Source: CAD feature listing. Evaluate the final solid. Frame: model axes, mm. A direction names the side the tool comes from. Round coordinates to 2 decimals unless told otherwise and drop trailing zeros. Order: outer loops, then holes, each group sorted by start corner. A loop starts at its lowest first (then second) coordinate and runs counter-clockwise, first axis right, second up. Notation, with made-up numbers: M 24,46 L 79,46 A11 cw 79,51 Z; hole C 2,36 d5. An arc over 180 degrees is marked long. Use one line per item in the form item = value. Start each with the question number.
Q1. Section D-D (y = -20). Return the cut outline in (x, z) (3 decimals).
Q2. Section B-B (z = -9.5). Return the cut outline in (x, y) (3 decimals).
Q3. Pull-direction query (X, two-part tool) for faces 3 (the cylindrical face through (12.024, -24.43, -0.86)), 4 (the cylindrical face through (6.8, -11.6, -1.9)), 5 (the flat face through (0, 0, -11)), 6 (the cylindrical face through (6.89, -18.99, 8.54)); classes: pulls with the +X half, pulls with the -X half, needs draft (parallel to the pull), parting line crosses it, or undercut.
Q4. Material intervals for probe 1 along Y at (x, z) = (8, 8.85); probe 2 along Y at (x, z) = (-8, 7.3); probe 3 along Y at (x, z) = (-8, 3), sorted ascending.
Q5. Contact query for flat-ended pins moving along their axis: pin 1 (1.5 mm diameter, centred on x = 8.5, y = -1, fed in from +Z); pin 2 (3.5 mm diameter, centred on x = 8, y = -10.7, fed in from +Z). Output: stop coordinate, or through.
Q6. Reachability of faces 1 (the flat face through (6, 8, 7)), 2 (the flat face through (0, -25, -1)) from +Z, -Z, +X, -X, +Y, -Y: full face, straight path, thin tool, end or side. Return the list, or none.
Q7. Section C-C (x = 8). Give the number of separate pieces and of enclosed holes in the cut face, plus the area to 3 significant figures.
Q8. Section A-A (y = 17.75). Return the cut outline in (x, z) (3 decimals), plus the area to 3 significant figures.
Autodesk Inventor part; units mm, degrees
ref_plane "YZ Plane" through (0, 0, 0) normal (1, 0, 0) x (0, 1, 0)
ref_plane "XZ Plane" through (0, 0, 0) normal (0, 1, 0) x (-1, 0, 0)
ref_plane "XY Plane" through (0, 0, 0) normal (0, 0, 1) x (1, 0, 0)
sketch "Эскиз1" plane through (0, 0, 0) normal (0, 0, 1) x (1, 0, 0)
  line L0 (-12.625, -25) -> (12.625, -25)
  line L1 (12.625, -25) -> (12.625, 25)
  line L2 (12.625, 25) -> (-12.625, 25)
  line L3 (-12.625, 25) -> (-12.625, -25)
  line L4 (-12.625, -25) -> (12.625, 25) construction
  line L5 (12.625, -25) -> (-12.625, 25) construction
  point P0 (0, 0)
  dimension "d0" = 25.25
  dimension "d1" = 50
extrude "Выдавливание1" add sketch "Эскиз1" along normal mid plane 22
fillet "Сопряжение1" radius 2 8 edges at (-12.625, -25, 0) (0, -25, 11) (-12.625, 0, 11) (12.625, 0, 11) (12.625, -25, 0) (0, 25, 11) (12.625, 25, 0) (-12.625, 25, 0)
sketch "Эскиз2" plane through (0, 0, 11) normal (0, 0, 1) x (1, 0, 0)
  circle A0 centre (-8, 17.75) radius 1.25
  circle A1 centre (8, 17.75) radius 1.25
  line L0 (-10.625, 23) -> (10.625, 23)
  point P0 (0, 0)
  dimension "d17" = 5.25
  dimension "d18" = 5.25
extrude "Выдавливание2" cut sketch "Эскиз2" against normal up to surface (22 mm away)
sketch "Эскиз3" plane through (0, 0, 11) normal (0, 0, 1) x (1, 0, 0)
  point P0 (0, 0)
sketch "Эскиз4" plane through (0, 0, 11) normal (0, 0, 1) x (1, 0, 0)
  circle A0 centre (8, 8) radius 1.5
  circle A1 centre (-8, 8) radius 1.5
  line L0 (-8, 8) -> (8, 8) construction
  circle A2 centre (-8, 17.75) radius 1.25 construction
  line L1 (-8, 17.75) -> (-8, 4.7032) construction
  line L2 (10.625, -23) -> (-10.625, -23) construction
  point P0 (0, 0)
  dimension "d7" = 3
  dimension "d8" = 16
  dimension "d16" = 9.75
extrude "Выдавливание3" cut sketch "Эскиз4" against normal up to surface (22 mm away)
sketch "Эскиз5" plane through (0, 0, 11) normal (0, 0, 1) x (1, 0, 0)
  circle A0 centre (8, 8) radius 1.5
  circle A1 centre (8, 8) radius 2.25
  circle A2 centre (-8, 8) radius 1.5
  line L0 (-8, 11.2332) -> (-5.2, 9.6166)
  line L1 (-5.2, 9.6166) -> (-5.2, 6.3834)
  line L2 (-5.2, 6.3834) -> (-8, 4.7668)
  line L3 (-8, 4.7668) -> (-10.8, 6.3834)
  line L4 (-10.8, 6.3834) -> (-10.8, 9.6166)
  line L5 (-10.8, 9.6166) -> (-8, 11.2332)
  point P0 (0, 0)
  dimension "d12" = 4.5
  dimension "d15" = 5.6
extrude "Выдавливание4" cut sketch "Эскиз5" against normal blind 4
sketch "Эскиз6" plane through (0, 0, 11) normal (0, 0, 1) x (1, 0, 0)
  circle A0 centre (-8, -1.3) radius 1.5
  circle A1 centre (8, -1.3) radius 1.5
  circle A2 centre (-8, -20) radius 1.5
  circle A3 centre (8, -20) radius 1.5
  line L0 (-8, -1.3) -> (-8, -20) construction
  line L1 (-8, -1.3) -> (8, -1.3) construction
  line L2 (-8, -20) -> (8, -20) construction
  line L3 (-10.625, -25) -> (10.625, -25)
  line L4 (10.625, -23) -> (-10.625, -23)
  line L5 (0, -23) -> (0, 23) construction
  line L6 (-10.625, 23) -> (10.625, 23)
  line L7 (0, 35) -> (0, -35)
  circle A4 centre (-8, 8) radius 1.5
  point P0 (0, 0)
  point P1 (0, -20)
  dimension "d19" = 3
  dimension "d20" = 16
  dimension "d21" = 16
  dimension "d23" = 5
  dimension "d40" = 9.3
extrude "Выдавливание5" cut sketch "Эскиз6" against normal blind 5 contours A0 | A1 | A2 | A3
sketch "Эскиз7" plane through (0, 0, 11) normal (0, 0, 1) x (1, 0, 0)
  circle A0 centre (-8, -20) radius 1.5
  circle A1 centre (-8, -1.3) radius 1.5
  line L0 (-8, -20) -> (-8, -1.3) construction
  circle A2 centre (8, -20) radius 1.5
  circle A3 centre (8, -1.3) radius 1.5
  line L1 (8, -20) -> (8, -1.3) construction
  circle A4 centre (8, -10.7) radius 2.25
  line L2 (-10.8, -9.0834) -> (-8, -7.4668)
  line L3 (-8, -7.4668) -> (-5.2, -9.0834)
  line L4 (-5.2, -9.0834) -> (-5.2, -12.3166)
  line L5 (-5.2, -12.3166) -> (-8, -13.9332)
  line L6 (-8, -13.9332) -> (-10.8, -12.3166)
  line L7 (-10.8, -12.3166) -> (-10.8, -9.0834)
  circle A5 centre (-8, -10.7) radius 1.5
  circle A6 centre (8, -10.7) radius 1.5
  point P0 (0, 0)
  dimension "d28" = 4.5
  dimension "d29" = 5.6
  dimension "d35" = 3
  dimension "d41" = 9.3
  dimension "d42" = 9.3
extrude "Выдавливание8" cut sketch "Эскиз7" against normal blind 4 contours A4 | L2 L3 L4 L5 L6 L7
sketch "Эскиз9" plane through (0, 0, 11) normal (0, 0, 1) x (1, 0, 0)
  circle A0 centre (-8, -10.7) radius 1.5
  circle A1 centre (8, -10.7) radius 1.5
  point P0 (0, 0)
extrude "Выдавливание9" cut sketch "Эскиз9" against normal up to surface (22 mm away)
properties part number "крепление петли хвоста"
Results list:
q1.outline = M -12.625,-11 L 12.625,-11 L 12.625,9 A2 ccw 10.625,11 L 9.5,11 L 9.5,6 L 6.5,6 L 6.5,11 L -6.5,11 L -6.5,6 L -9.5,6 L -9.5,11 L -10.625,11 A2 ccw -12.625,9 Z
q2.outline = M -12.625,-23 A2 ccw -10.625,-25 L 10.625,-25 A2 ccw 12.625,-23 L 12.625,23 A2 ccw 10.625,25 L -10.625,25 A2 ccw -12.625,23 Z; hole C -8,-10.7 d3; hole C -8,8 d3; hole C -8,17.75 d2.5; hole C 8,-10.7 d3; hole C 8,8 d3; hole C 8,17.75 d2.5
q3.face_3 = pulls with the +X half
q3.face_4 = undercut
q3.face_5 = needs draft
q3.face_6 = undercut
q4.probe_1 = -25 to -21.5, -18.5 to -12.95, -8.45 to -2.8, 0.2 to 5.75, 10.25 to 16.5, 19 to 25
q4.probe_2 = -25 to -21.5, -18.5 to -13.93, -7.47 to -2.8, 0.2 to 4.77, 11.23 to 16.5, 19 to 25
q4.probe_3 = -25 to -12.2, -9.2 to 6.5, 9.5 to 16.5, 19 to 25
q5.pin_1 = 6
q5.pin_2 = 7
q6.face_1 = +Z
q6.face_2 = +Z, -Z, +X, -X, -Y
q7.separate_pieces = 4
q7.enclosed_holes = 0
q7.area = 869 mm2
q8.outline = M -12.625,-11 L -9.25,-11 L -9.25,11 L -10.625,11 A2 ccw -12.625,9 Z; M -6.75,-11 L 6.75,-11 L 6.75,11 L -6.75,11 Z; M 9.25,-11 L 12.625,-11 L 12.625,9 A2 ccw 10.625,11 L 9.25,11 Z
q8.area = 444 mm2
